Build history of the part. All positions in model axes, mm. Face numbers are marked on the shaded views. A direction names the side the tool comes from. Round coordinates to 2 decimals unless told otherwise and drop trailing zeros. Write each loop counter-clockwise with the first axis right and the second up, starting at its lowest first coordinate (ties: lowest second). Pieces come first, ordered by that corner, then holes. Notation, with made-up numbers: (53, 41.5) -> (80, 41.5) arc R28 ccw to (80, 61.5) -> close; hole circle Ø1 at (55.25, 87.5). An arc over 180 degrees is marked (long way). Answer in a Markdown table with one row per item. Add a question column.
from build123d import *

# Parameters (mm, degrees)
F0_W     = 127.737302
F0_H     = 90.112857
F1_DEPTH = 25.4
F2_W     = 11.786669
F2_H     = 10.160922
F2_W_2   = 18.289661
F2_H_2   = 11.380233
F2_W_3   = 15.851038
F2_H_3   = 11.786668
F2_W_4   = 19.915408
F2_H_4   = 12.599544
F2_W_5   = 18.696092
F2_H_5   = 13.412416
F2_W_6   = 12.193104
F2_H_6   = 9.754487
F3_DEPTH = 25.4
F4_R     = 5.08


with BuildPart() as f1:
    # F0 (on Top) → F1 (new body)
    with BuildSketch(Plane.XY):
        with Locations((8.128738, -7.548112)):
            Rectangle(F0_W, F0_H)
    extrude(amount=F1_DEPTH)

    # F2 (on face) → F3 (cut)
    with BuildSketch(Plane.XY.offset(25.4)):
        with Locations((0.609656, 15.444601)):
            Rectangle(F2_W, F2_H)
        with Locations((35.563227, 14.42851)):
            Rectangle(F2_W_2, F2_H_2)
        with Locations((-24.182993, -26.418396)):
            Rectangle(F2_W_3, F2_H_3)
        with Locations((9.957704, -26.418398)):
            Rectangle(F2_W_4, F2_H_4)
        with Locations((44.301618, -30.482765)):
            Rectangle(F2_W_5, F2_H_5)
        with Locations((-31.702076, 17.273567)):
            Rectangle(F2_W_6, F2_H_6)
    extrude(amount=-F3_DEPTH, mode=Mode.SUBTRACT)

    # F4
    f4_edges = [f1.edges().sort_by_distance(p)[0] for p in [
        (-31.702076, 22.150811, 25.4),
        (-37.798628, 17.273568, 25.4),
        (-31.702076, 12.396324, 25.4),
        (-25.605524, 17.273568, 25.4),
        (0.609656, 20.525062, 25.4),
        (6.502991, 15.444601, 25.4),
        (0.609656, 10.36414, 25.4),
        (-5.283678, 15.444601, 25.4),
        (35.563228, 20.118626, 25.4),
        (35.563228, 8.738393, 25.4),
        (26.418397, 14.428509, 25.4),
        (44.708058, 14.428509, 25.4),
        (19.915408, -26.418398, 25.4),
        (9.957704, -32.71817, 25.4),
        (0, -26.418398, 25.4),
        (9.957704, -20.118626, 25.4),
        (34.953572, -30.482765, 25.4),
        (44.301618, -23.776557, 25.4),
        (53.649664, -30.482765, 25.4),
        (44.301618, -37.188973, 25.4),
        (-32.108512, -26.418396, 25.4),
        (-24.182993, -20.525062, 25.4),
        (-24.182993, -32.31173, 25.4),
        (-16.257474, -26.418396, 25.4),
        (8.128738, 37.508316, 25.4),
        (71.997389, -7.548112, 25.4),
        (8.128738, -52.604541, 25.4),
        (-55.739913, -7.548112, 25.4),
    ]]
    fillet(f4_edges, radius=F4_R)


solid = f1.part
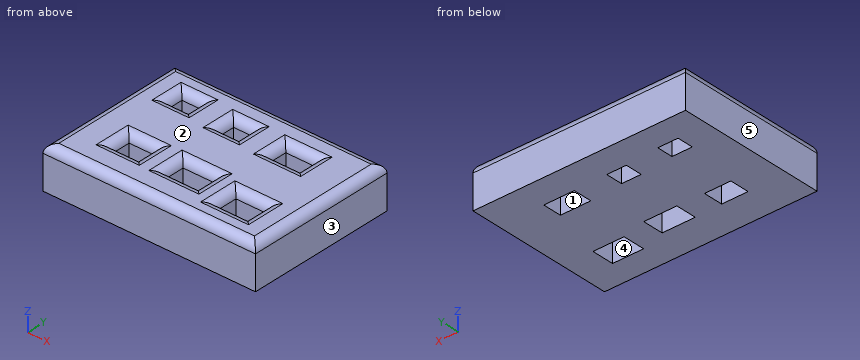
(1) Saw through at B-B (z = 9). List the corners of the cut face in (x, y).
(2) Saw through at A-A (x = -33.5). List the corners of the cut face in (y, z).
(3) Mould opens along X. For the marked faces 1, 2 and 3 say: pulls with the +X half, pulls with the -X half, needs draft (parallel to the pull), parting line crosses it, or undercut.
(4) Probe line 1 along X through (y, z) = (14, 19.5); line 2 along X through (y, z) = (-31.5, 9.5); line 3 along Y through (x, z) = (3, 4). List the from-to ranges inside material, lowest first.
(5) Saw through at C-C (y = -35.5). List the corners of the cut face in (x, z), plus the area to 3 significant figures.
(6) Saw through at D-D (z = 23). List the corners of the cut face in (x, y), plus the area to 3 significant figures.
(7) Which spindle directions (+Z, -Z, +X, -X, +Y, -Y) get a long thin tool onto all of the face, cutting with end or side? Do the marked faces 4 and 5. Say none if no direction does.
Answer sheet:
| question | item | result |
|---|---|---|
| 1 | outline | (-55.74, -52.6) -> (72, -52.6) -> (72, 37.51) -> (-55.74, 37.51) -> close; hole (-37.8, 12.4) -> (-25.61, 12.4) -> (-25.61, 22.15) -> (-37.8, 22.15) -> close; hole (-32.11, -32.31) -> (-16.26, -32.31) -> (-16.26, -20.53) -> (-32.11, -20.53) -> close; hole (-5.28, 10.36) -> (6.5, 10.36) -> (6.5, 20.53) -> (-5.28, 20.53) -> close; hole (0, -32.72) -> (19.92, -32.72) -> (19.92, -20.12) -> (0, -20.12) -> close; hole (26.42, 8.74) -> (44.71, 8.74) -> (44.71, 20.12) -> (26.42, 20.12) -> close; hole (34.95, -37.19) -> (53.65, -37.19) -> (53.65, -23.78) -> (34.95, -23.78) -> close |
| 2 | outline | (-52.6, 0) -> (12.4, 0) -> (12.4, 20.32) arc R5.08 ccw to (7.32, 25.4) -> (-15.45, 25.4) arc R5.08 ccw to (-19.13, 23.81) -> (-33.7, 23.81) arc R5.08 ccw to (-37.39, 25.4) -> (-47.52, 25.4) arc R5.08 ccw to (-52.6, 20.32) -> close; (22.15, 0) -> (37.51, 0) -> (37.51, 20.32) arc R5.08 ccw to (32.43, 25.4) -> (27.23, 25.4) arc R5.08 ccw to (22.15, 20.32) -> close |
| 3 | face 1 | undercut |
| 3 | face 2 | needs draft |
| 3 | face 3 | pulls with the +X half |
| 4 | line 1 | x = -55.74 to -37.8, -25.61 to -5.28, 6.5 to 26.42, 44.71 to 72 |
| 4 | line 2 | x = -55.74 to -32.11, -16.26 to 0, 19.92 to 34.95, 53.65 to 72 |
| 4 | line 3 | y = -52.6 to -32.72, -20.12 to 10.36, 20.53 to 37.51 |
| 5 | outline | (-55.74, 0) -> (34.95, 0) -> (34.95, 20.32) arc R5.08 ccw to (29.87, 25.4) -> (25, 25.4) arc R5.08 ccw to (22.7, 24.85) -> (-2.78, 24.85) arc R5.08 ccw to (-5.08, 25.4) -> (-11.18, 25.4) arc R5.08 ccw to (-13.07, 25.03) -> (-35.3, 25.03) arc R5.08 ccw to (-37.19, 25.4) -> (-50.66, 25.4) arc R5.08 ccw to (-55.74, 20.32) -> close; (53.65, 0) -> (72, 0) -> (72, 20.32) arc R5.08 ccw to (66.92, 25.4) -> (58.73, 25.4) arc R5.08 ccw to (53.65, 20.32) -> close |
| 5 | area | 2,720 mm² |
| 6 | outline | (-54.98, -51.84) -> (71.23, -51.84) -> (71.23, 36.74) -> (-54.98, 36.74) -> close; hole (-38.56, 11.63) -> (-24.84, 11.63) -> (-24.84, 22.92) -> (-38.56, 22.92) -> close; hole (-32.87, -33.08) -> (-15.49, -33.08) -> (-15.49, -19.76) -> (-32.87, -19.76) -> close; hole (-6.05, 9.6) -> (7.27, 9.6) -> (7.27, 21.29) -> (-6.05, 21.29) -> close; hole (-0.76, -33.48) -> (20.68, -33.48) -> (20.68, -19.35) -> (-0.76, -19.35) -> close; hole (25.65, 7.97) -> (45.47, 7.97) -> (45.47, 20.88) -> (25.65, 20.88) -> close; hole (34.19, -37.95) -> (54.41, -37.95) -> (54.41, -23.01) -> (34.19, -23.01) -> close |
| 6 | area | 9,780 mm² |
| 7 | face 4 | +Z, -Z |
| 7 | face 5 | +Z, -Z, -X, +Y, -Y |
